from build123d import *

# Parameters (mm, degrees)
SKETCH1_W           = 50
SKETCH1_H           = 50
BOSS_EXTRUDE1_DEPTH = 50
SKETCH4_OUTSIDE_W   = 69.32
SKETCH4_OUTSIDE_H   = 69.32
CUT_EXTRUDE3_DEPTH  = 62.23724357
SKETCH5_OUTSIDE_W   = 69.32
SKETCH5_OUTSIDE_H   = 69.32
CUT_EXTRUDE4_DEPTH  = 62.23724357
SKETCH6_OUTSIDE_W   = 69.32
SKETCH6_OUTSIDE_H   = 69.32
CUT_EXTRUDE5_DEPTH  = 62.23724357
SKETCH7_OUTSIDE_W   = 69.32
SKETCH7_OUTSIDE_H   = 69.32
CUT_EXTRUDE6_DEPTH  = 62.23724357


with BuildPart() as part:
    # Sketch1 → Boss-Extrude1 (new body)
    with BuildSketch(Plane(origin=(0, 0, 0), x_dir=(1, 0, 0), z_dir=(0, 1, 0))):
        Rectangle(SKETCH1_W, SKETCH1_H)
    extrude(amount=BOSS_EXTRUDE1_DEPTH)

    # Sketch4 outside → Cut-Extrude3 (cut, through all)
    with BuildSketch(Plane(origin=(0, 0, 0), x_dir=(0, 0, -1), z_dir=(1, 0, 0))):
        with Locations((0, 25)):
            Rectangle(SKETCH4_OUTSIDE_W, SKETCH4_OUTSIDE_H)
        Polygon((-25, 0), (0, 50), (25, 0), align=None, mode=Mode.SUBTRACT)
    extrude(amount=-CUT_EXTRUDE3_DEPTH, mode=Mode.SUBTRACT)

    # Sketch5 outside → Cut-Extrude4 (cut, through all)
    with BuildSketch(Plane(origin=(0, 0, 0), x_dir=(0, 0, -1), z_dir=(1, 0, 0))):
        with Locations((0, 25)):
            Rectangle(SKETCH5_OUTSIDE_W, SKETCH5_OUTSIDE_H)
        Polygon((-25, 0), (0, 50), (25, 0), align=None, mode=Mode.SUBTRACT)
    extrude(amount=CUT_EXTRUDE4_DEPTH, mode=Mode.SUBTRACT)

    # Sketch6 outside → Cut-Extrude5 (cut, through all)
    with BuildSketch(Plane.XY):
        with Locations((0, 25)):
            Rectangle(SKETCH6_OUTSIDE_W, SKETCH6_OUTSIDE_H)
        Polygon((-25, 0), (0, 50), (25, 0), align=None, mode=Mode.SUBTRACT)
    extrude(amount=-CUT_EXTRUDE5_DEPTH, mode=Mode.SUBTRACT)

    # Sketch7 outside → Cut-Extrude6 (cut, through all)
    with BuildSketch(Plane.XY):
        with Locations((0, 25)):
            Rectangle(SKETCH7_OUTSIDE_W, SKETCH7_OUTSIDE_H)
        Polygon((-25, 0), (0, 50), (25, 0), align=None, mode=Mode.SUBTRACT)
    extrude(amount=CUT_EXTRUDE6_DEPTH, mode=Mode.SUBTRACT)


solid = part.part
The listing builds one solid part. Answer for the finished solid, in the listing's coordinates (mm). Give positions to 0.01 mm unless a question says otherwise; leave off trailing zeros. Write each loop counter-clockwise with the first axis right and the second up, starting at its lowest first coordinate (ties: lowest second). Pieces come first, ordered by that corner, then holes.
Item 1: Section B-B, the plane z = 5 is taken. Write down the section's boundary in (x, y), plus the area to 3 significant figures.
Item 2: Flat-ended cylindrical pins translate along their axes: P1, Ø10, axis at y = 41.5, z = -11.5, coming from the -X side (3 decimals); P2, Ø2, axis at x = 4.5, y = 38.5, coming from the -Z side; P3, Ø6, axis at x = -9.5, z = -11.5, coming from the +Y side; P4, Ø10, axis at x = -2.5, z = -15.5, coming from the +Y side. Find the tip coordinate at first contact, or state that the pin passes through.
Item 3: Section A-A, the plane y = 30 is taken. Write down the section's boundary in (x, z).
Item 4: Find the intervals of material crossed by line 1 along Y through (x, z) = (-11, 11); line 2 along Y through (x, z) = (-4, -2.5); line 3 along Z through (x, y) = (-0.5, 23), in increasing order.
Completed:
1. outline: (-25, 0) - (25, 0) - (5, 40) - (-5, 40) - close
1. area: 1,200 mm2
2. P1: passes through
2. P2: stops at z = -6.25
2. P3: stops at y = 32.74
2. P4: stops at y = 29
3. outline: (-10, -10) - (10, -10) - (10, 10) - (-10, 10) - close
4. line 1: y = 0 to 28
4. line 2: y = 0 to 42
4. line 3: z = -13.5 to 13.5
